from build123d import *

# Parameters (mm, degrees)
OUTLINE_DEPTH        = 40
OUTLINE_DEPTH_BACK   = 40
SKETCH1_W            = 18.25
SKETCH1_H            = 40
SKETCH2_W            = 40
SKETCH2_H            = 80
EXTRUSION15_DEPTH    = 6
CAMERA_MOUNT_D       = 24.5364
SKETCH5_R            = 17.5
SKETCH5_R_2          = 12.268
EXTRUSION19_DEPTH    = 5.9562
CUT_EXTRUDE1_START   = -3
SKETCH10_W           = 80
SKETCH10_H           = 80
SKETCH10_R           = 17.5
CUT_EXTRUDE1_DEPTH   = 3
SKETCH6_W            = 80
SKETCH6_H            = 40
EXTRUSION21_DEPTH    = 6
SKETCH7_W            = 60
SKETCH7_H            = 60
EXTRUSION22_DEPTH    = 9
FILLET4_R            = 3.175
HOLE7_D              = 3.3
HOLE7_DEPTH          = 12
HOLE7_TIP            = 0.991420021
SKETCH11_OUTSIDE_W   = 105.14
SKETCH11_OUTSIDE_H   = 105.14
SKETCH11_OUTSIDE_W_2 = 74
SKETCH11_OUTSIDE_H_2 = 74
CUT_EXTRUDE2_DEPTH   = 59.588074725
CUT_EXTRUDE3_START   = -3
CUT_EXTRUDE3_DEPTH   = 3


with BuildPart() as part:
    # Sketch1 → Outline (new, two sides: drawn at the far end of the back side and taken through both)
    with BuildSketch(Plane.YZ.offset(-OUTLINE_DEPTH_BACK)):
        Polygon((18.25, 40), (5.33, 40), (0, 40), (0, 0), (18.25, 0), align=None)
        with Locations((9.125, -20)):
            Rectangle(SKETCH1_W, SKETCH1_H)
    extrude(amount=OUTLINE_DEPTH + OUTLINE_DEPTH_BACK)

    # Sketch2 → Extrusion15 (cut)
    with BuildSketch(Plane.XZ):
        Rectangle(SKETCH2_W, SKETCH2_H)
    extrude(amount=-EXTRUSION15_DEPTH, mode=Mode.SUBTRACT)

    # Camera mount (through all)
    with Locations(Plane(origin=(0, 18.25, 0), x_dir=(1, 0, 0), z_dir=(0, 1, 0))):
        with Locations((0, 0)):
            Hole(CAMERA_MOUNT_D / 2)

    # Sketch5 → Extrusion19 (add)
    with BuildSketch(Plane(origin=(0, 18.25, 0), x_dir=(-1, 0, 0), z_dir=(0, 1, 0))):
        with Locations(Location((0, 0, 0), (0, 0, 90))):
            Circle(SKETCH5_R)
        with Locations(Location((0, 0, 0), (0, 0, 90))):
            Circle(SKETCH5_R_2, mode=Mode.SUBTRACT)
    extrude(amount=EXTRUSION19_DEPTH)

    # Sketch10 → Cut-Extrude1 (cut)
    with BuildSketch(Plane(origin=(0, 18.25, 0), x_dir=(1, 0, 0), z_dir=(0, 1, 0)).offset(CUT_EXTRUDE1_START)):
        Rectangle(SKETCH10_W, SKETCH10_H)
        with Locations(Location((0, 0, 0), (0, 0, 270))):
            Circle(SKETCH10_R, mode=Mode.SUBTRACT)
    extrude(amount=CUT_EXTRUDE1_DEPTH, mode=Mode.SUBTRACT)

    # Sketch6 → Extrusion21 (cut)
    with BuildSketch(Plane.XZ):
        Rectangle(SKETCH6_W, SKETCH6_H)
    extrude(amount=-EXTRUSION21_DEPTH, mode=Mode.SUBTRACT)

    # Sketch7 → Extrusion22 (cut)
    with BuildSketch(Plane.XZ):
        Rectangle(SKETCH7_W, SKETCH7_H)
    extrude(amount=-EXTRUSION22_DEPTH, mode=Mode.SUBTRACT)

    # Fillet4
    fillet4_edges = [part.edges().sort_by_distance(p)[0] for p in [
        (-30, 4.5, 30),
        (30, 4.5, -30),
        (30, 4.5, 30),
        (-30, 4.5, -30),
        (0, 15.25, -17.5),
    ]]
    fillet(fillet4_edges, radius=FILLET4_R)

    # Hole7
    with Locations(Plane(origin=(0, 0, 0), x_dir=(-1, 0, 0), z_dir=(0, -1, 0))):
        with Locations((32.5, 32.5), (-32.5, 32.5), (-32.5, -32.5), (32.5, -32.5)):
            Hole(HOLE7_D / 2, depth=HOLE7_DEPTH)
            with Locations((0, 0, -(HOLE7_DEPTH + HOLE7_TIP / 2))):  # 118° drill point
                Cone(0, HOLE7_D / 2, HOLE7_TIP, mode=Mode.SUBTRACT)

    # Sketch11 outside → Cut-Extrude2 (cut, through all)
    with BuildSketch(Plane(origin=(0, 15.25, 0), x_dir=(1, 0, 0), z_dir=(0, 1, 0))):
        Rectangle(SKETCH11_OUTSIDE_W, SKETCH11_OUTSIDE_H)
        Rectangle(SKETCH11_OUTSIDE_W_2, SKETCH11_OUTSIDE_H_2, mode=Mode.SUBTRACT)
    extrude(amount=-CUT_EXTRUDE2_DEPTH, mode=Mode.SUBTRACT)

    # Sketch13 → Cut-Extrude3 (cut)
    with BuildSketch(Plane.XZ.offset(-9).offset(CUT_EXTRUDE3_START)):
        with BuildLine():
            Line((26.825, 30), (-26.825, 30))
            ThreePointArc((-26.825, 30), (-29.07006403, 29.07006403), (-30, 26.825))
            Line((-30, 26.825), (-30, -26.825))
            ThreePointArc((-30, -26.825), (-29.07006403, -29.07006403), (-26.825, -30))
            Line((-26.825, -30), (26.825, -30))
            ThreePointArc((26.825, -30), (29.07006403, -29.07006403), (30, -26.825))
            Line((30, -26.825), (30, 26.825))
            ThreePointArc((30, 26.825), (29.07006403, 29.07006403), (26.825, 30))
        make_face()
    extrude(amount=CUT_EXTRUDE3_DEPTH, mode=Mode.SUBTRACT)


solid = part.part
Read the model definition and answer for the solid it produces. Units are mm, in the model's axes. A direction names the side the tool comes from. Give positions to 0.01 mm unless a question says otherwise; leave off trailing zeros. Write each loop counter-clockwise with the first axis right and the second up, starting at its lowest first coordinate (ties: lowest second). Pieces come first, ordered by that corner, then holes. Notation, with made-up numbers: M 36.5,17 L 57.5,17 A21 ccw 57.5,29 Z; hole C 22.25,-2.75 d10. An arc over 180 degrees is marked long. One line per item, written item: value. Start each with the question number.
(1) Find section A-A (y = 2). Give the number of separate pieces and of enclosed holes in the cut face, plus the area to 3 significant figures.
(2) Determine the mould class of faces 1 (the flat face through (-17, 15.25, -17)), 2 (the flat face through (0, 9, 30)), 3 (the flat face through (-34, 3, 20)) for opening direction Z: pulls with the +Z half, pulls with the -Z half, needs draft (parallel to the pull), parting line crosses it, or undercut.
(3) Find section D-D (y = 21). Determine the outline of the cut face in (x, z), plus the area to 3 significant figures.
(4) A tool of negligible diameter and unlimited length cuts with its end or side. For faces 4 (the flat face through (-20, 3, -34)), 5 (the flat face through (33, 3, -20)), 6 (the cylindrical face through (-32.715, 6.084, 30.864)), from which of +Z, -Z, +X, -X, +Y, -Y can it reach the whole face along a straight path? Write none if from no direction.
(5) Flat-ended cylindrical pins translate along their axes: pin 1 Ø2 at (x, z) = (33.5, -3) entering from -Y; pin 2 Ø4 at (y, z) = (18, 4) entering from -X; pin 3 Ø3 at (x, z) = (-28, -25.5) entering from -Y. Find the tip coordinate at first contact, or state that the pin passes through.
(6) Find the intervals of material crossed by line 1 (X direction, y = 8.25, z = 32.5); line 2 (Z direction, x = 32.5, y = 4.5); line 3 (Z direction, x = -13, y = 8.5), in increasing order.
Results below:
1. separate pieces: 4
1. enclosed holes: 4
1. area: 730 mm^2
2. face 1: needs draft
2. face 2: undercut
2. face 3: undercut
3. outline: C 0,0 d35; hole C 0,0 d24.54
3. area: 489 mm^2
4. face 4: +Z, -Z, -Y
4. face 5: +X, -X, -Y
4. face 6: -Y
5. pin 1: stops at y = 6
5. pin 2: stops at x = -18.23
5. pin 3: stops at y = 12
6. line 1: x = -37 to -34.15, -30.85 to 30.85, 34.15 to 37
6. line 2: z = -37 to -34.15, -30.85 to -20, 20 to 30.85, 34.15 to 37
6. line 3: z = -37 to -30, 30 to 37
